For this review, use the dimensioned drawing (mm, ordinates from the lowest corner) and the shaded views. Give positions to 0.01 mm unless a question says otherwise; leave off trailing zeros. Write each loop counter-clockwise with the first axis right and the second up, starting at its lowest first coordinate (ties: lowest second). Pieces come first, ordered by that corner, then holes. Notation, with made-up numbers: (9, 20) - (52, 20) arc R8 cw to (52, 31) - close; hole circle Ø1 at (62, 60). An arc over 180 degrees is marked (long way). Use a Markdown table: item, result. Add a question column.
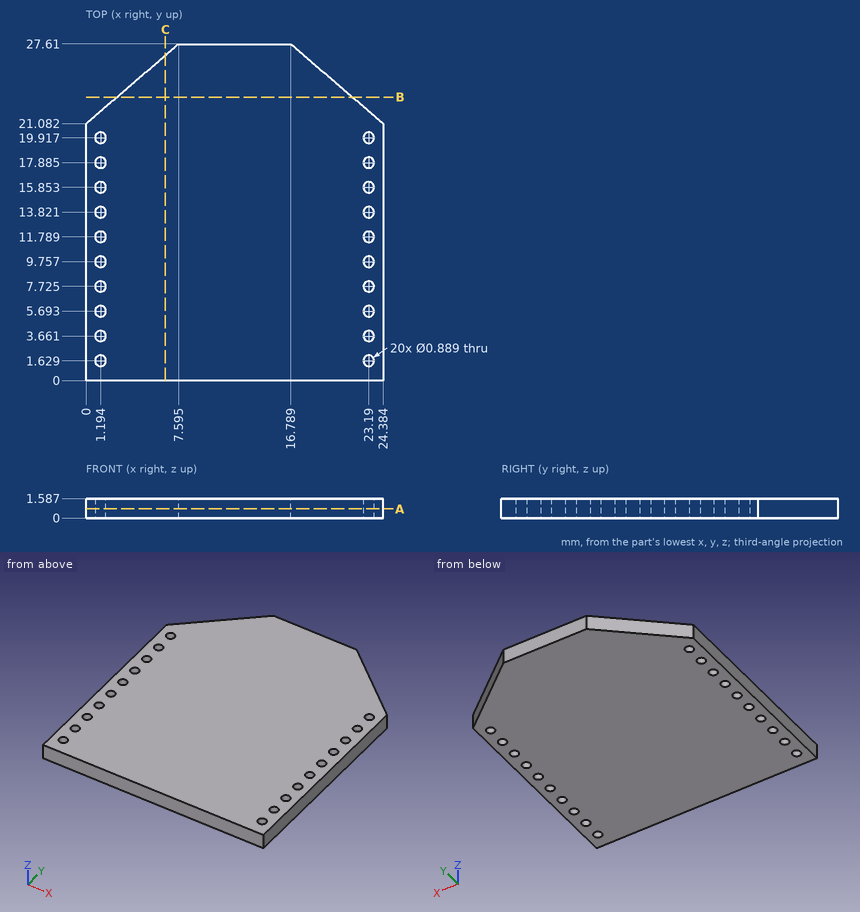
(1) For line 1 along X through (y, z) = (10, 1.05) (1 decimal); line 2 along Y through (x, z) = (3.5, 0.75); line 3 along X through (y, z) = (22, 0.55) (1 decimal), list the stretches that pass through material, from the lowest coordinate up.
(2) Add section B-B (y = 23.25). State the section outline as (x, z) points.
(3) Add section A-A (z = 0.75). Count the separate pieces of the cut face and the enclosed holes in it, and give its area (3 significant figures).
(4) Add section C-C (x = 6.5). State the section outline as (y, z) points.
Answers follow:
| question | item | result |
|---|---|---|
| 1 | line 1 | 0 to 0.8, 1.6 to 22.8, 23.6 to 24.4 |
| 1 | line 2 | 0 to 24.09 |
| 1 | line 3 | 1.1 to 23.3 |
| 2 | outline | (2.52, 0) - (21.86, 0) - (21.86, 1.59) - (2.52, 1.59) - close |
| 3 | separate pieces | 1 |
| 3 | enclosed holes | 20 |
| 3 | area | 611 mm^2 |
| 4 | outline | (0, 0) - (26.67, 0) - (26.67, 1.59) - (0, 1.59) - close |
